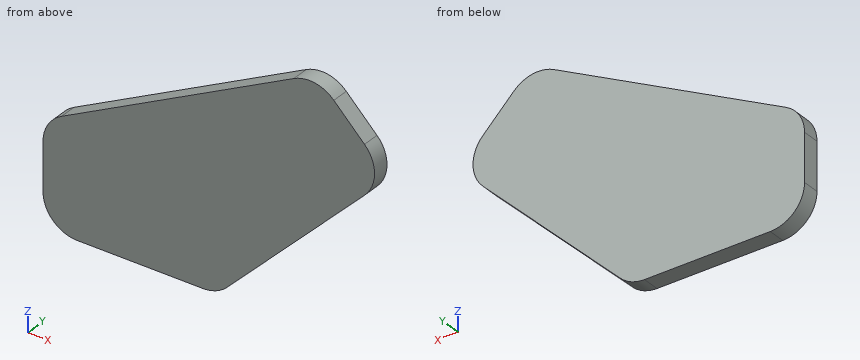
Autodesk Inventor part; units mm, degrees
ref_plane "YZ Plane" through (0, 0, 0) normal (1, 0, 0) x (0, 1, 0)
ref_plane "XZ Plane" through (0, 0, 0) normal (0, 1, 0) x (-1, 0, 0)
ref_plane "XY Plane" through (0, 0, 0) normal (0, 0, 1) x (1, 0, 0)
sketch "Sketch1" plane through (0, 0, 0) normal (0, 1, 0) x (-1, 0, 0)
  line L0 (0, 25) -> (0, -25)
  line L1 (0, 25) -> (-59.2893, 25) construction
  line L2 (-59.2893, 25) -> (-143.6396, 109.3503) construction
  line L3 (-143.6396, 109.3503) -> (-178.9949, 73.9949)
  line L4 (-178.9949, 73.9949) -> (-80, -25)
  line L5 (-80, -25) -> (0, -25)
  line L6 (-25, 25) -> (-25, -25)
  line L7 (-97.6777, 63.3883) -> (-133.033, 28.033)
  line L8 (-25, 15) -> (-104.7487, 56.3173)
  line L9 (-25, -15) -> (-75.8579, -15)
  line L10 (-75.8579, -15) -> (-125.9619, 35.1041)
  point P0 (0, 0)
  point P1 (0, 0)
  dimension "d0" = 50
  dimension "d1" = 80
  dimension "d2" = 135
  dimension "d3" = 140
  dimension "d4" = 50
  dimension "d37" = 25
  dimension "d38" = 65
  dimension "d39" = 10
  dimension "d40" = 10
  dimension "d41" = 10
  dimension "d42" = 10
extrude "Plate1" add sketch "Sketch1" along normal blind 5 contours L7 L8 L6 L9 L10
fillet "Corner Round1" radius 10 5 edges at (25, 2.5, -15) (25, 2.5, 15) (104.7487, 2.5, 56.3173) (125.9619, 2.5, 35.1041) (75.8579, 2.5, -15)
equation "\"d4\" = d0"
equation "\"d40\" = d39"
equation "\"d41\" = d39"
equation "\"d42\" = d41"
equation "\"d5\" = Thickness"
equation "\"BendRadius\" = Thickness"
equation "\"BendReliefWidth\" = Thickness"
equation "\"BendReliefDepth\" = 0.5 * Thickness"
equation "\"TransitionRadius\" = BendRadius"
equation "\"JacobiRadiusSize\" = BendRadius"
equation "\"GapSize\" = Thickness"
properties part number "PWTR-0089" material "Stainless Steel"
Model file for the job. Use its own axes, mm. Coordinates: 2 decimals unless noted, no trailing zeros. Loops run counter-clockwise (first coordinate to the right, second up) from the corner with the lowest first, then second, coordinate; pieces in that order, holes last. Notation, with made-up numbers: (25.5, 85.25) - (49.5, 85.25) arc R23 cw to (49.5, 97.25) - close; hole circle Ø6 at (-35, 88). An arc over 180 degrees is marked (long way). Write item = value, one per line. Start each with the question number.
Item 1: Wall check: probe 1 along X at (y, z) = (2.7, 35); probe 2 along X at (y, z) = (0.4, 9); probe 3 along Z at (x, y) = (115.5, 4.4). Give the ranges that are in metal, low to high. Write a range as [from, to].
Item 2: Saw through at B-B, the plane z = 16.5. List the corners of the cut face in (x, y).
Item 3: Drop flat-ended pins along their axis: pin 1 Ø1.5 at (y, z) = (1, 14) entering from -X; pin 2 Ø2 at (y, z) = (4, 39.5) entering from +X; pin 3 Ø1 at (x, z) = (95.5, 2) entering from +Y; pin 4 Ø2 at (x, y) = (36.5, 2.5) entering from +Z. Give the stop position or say it passes through.
Item 4: Saw through at C-C, the plane x = 96. List the corners of the cut face in (y, z), then the cut area to 3 significant figures.
Item 5: Saw through at A-A, the plane y = 3. List the corners of the cut face in (x, z).
Answers:
q1.probe_1 = [63.6, 121.82]
q1.probe_2 = [25, 99.86]
q1.probe_3 = [24.64, 45.57]
q2.outline = (28.48, 0) - (107.36, 0) - (107.36, 5) - (28.48, 5) - close
q3.pin_1 = 25.99
q3.pin_2 = 121.23
q3.pin_3 = through
q3.pin_4 = 21.48
q4.outline = (0, 5.14) - (5, 5.14) - (5, 51.78) - (0, 51.78) - close
q4.area = 233 mm2
q5.outline = (25, -5) arc R10 ccw to (35, -15) - (71.72, -15) arc R10 ccw to (78.79, -12.07) - (118.89, 28.03) arc R10 ccw to (118.89, 42.18) - (109.92, 51.14) arc R10 ccw to (98.25, 52.95) - (30.4, 17.8) arc R10 ccw to (25, 8.92) - close
